Source: CAD feature listing. Evaluate the final solid. Frame: model axes, mm. Face numbers are marked on the shaded views. Coordinates: 2 decimals unless noted, no trailing zeros. Loops run counter-clockwise (first coordinate to the right, second up) from the corner with the lowest first, then second, coordinate; pieces in that order, holes last.
from build123d import *

# Parameters (mm, degrees)
SKETCH1_W                        = 234.95
SKETCH1_H                        = 76.2
EXTRUDE1_DEPTH                   = 12.7
F_1_2_CLEARANCE_HOLE1_AT_2_COUNT = 2
F_1_2_CLEARANCE_HOLE1_AT_2_PITCH = 44.45
F_1_2_CLEARANCE_HOLE1_AT_3_COUNT = 2
F_1_2_CLEARANCE_HOLE1_AT_3_PITCH = 203.2
F_1_2_CLEARANCE_HOLE1_AT_4_COUNT = 2
F_1_2_CLEARANCE_HOLE1_AT_4_PITCH = 208.004909798
SKETCH6_W                        = 171.45
SKETCH6_H                        = 76.2
CUT_EXTRUDE1_DEPTH               = 1.016
F_1_4_20_TAPPED_HOLE1_AT_2_COUNT = 2
F_1_4_20_TAPPED_HOLE1_AT_2_PITCH = 63.5
F_1_4_20_TAPPED_HOLE1_AT_3_COUNT = 2
F_1_4_20_TAPPED_HOLE1_AT_3_PITCH = 127


with BuildPart() as part:
    # Sketch1 → Extrude1 (new body)
    with BuildSketch(Plane.XY):
        Rectangle(SKETCH1_W, SKETCH1_H)
    extrude(amount=EXTRUDE1_DEPTH)

    # Sketch2 → 1/2 Clearance Hole1 (revolve, cut)
    with BuildSketch(Plane(origin=(-101.6, 22.225, 12.7), x_dir=(0, -1, 0), z_dir=(1, 0, 0))):
        Polygon((0, 0), (0, 12.7), (10.16, 12.7), (9.525, 11.969516061), (9.525, 0.730483939), (10.16, 0), align=None)
    f_1_2_clearance_hole1 = revolve(axis=Axis((-101.6, 22.225, 19.05), (0, 0, -1)), mode=Mode.SUBTRACT)

    # 1/2 Clearance Hole1 at 2: 1/2 Clearance Hole1 ×2
    with Locations(*[(0, -i * F_1_2_CLEARANCE_HOLE1_AT_2_PITCH, 0) for i in range(1, F_1_2_CLEARANCE_HOLE1_AT_2_COUNT)]):
        add(f_1_2_clearance_hole1, mode=Mode.SUBTRACT)

    # 1/2 Clearance Hole1 at 3: 1/2 Clearance Hole1 ×2
    with Locations(*[(i * F_1_2_CLEARANCE_HOLE1_AT_3_PITCH, 0, 0) for i in range(1, F_1_2_CLEARANCE_HOLE1_AT_3_COUNT)]):
        add(f_1_2_clearance_hole1, mode=Mode.SUBTRACT)

    # 1/2 Clearance Hole1 at 4: 1/2 Clearance Hole1 ×2
    with Locations(*[Vector(0.976900017, -0.213696879, 0) * (i * F_1_2_CLEARANCE_HOLE1_AT_4_PITCH) for i in range(1, F_1_2_CLEARANCE_HOLE1_AT_4_COUNT)]):
        add(f_1_2_clearance_hole1, mode=Mode.SUBTRACT)

    # Sketch6 → Cut-Extrude1 (cut)
    with BuildSketch(Plane(origin=(0, 0, 0), x_dir=(-1, 0, 0), z_dir=(0, 0, -1))):
        Rectangle(SKETCH6_W, SKETCH6_H)
    extrude(amount=-CUT_EXTRUDE1_DEPTH, mode=Mode.SUBTRACT)

    # Sketch4 → 1/4-20 Tapped Hole1 (revolve, cut)
    with BuildSketch(Plane(origin=(-63.5, 0, 12.7), x_dir=(0, -1, 0), z_dir=(1, 0, 0))):
        Polygon((0, 0), (0, 11.684), (3.81, 11.684), (2.5527, 10.237641802), (2.5527, 1.446358198), (3.81, 0), align=None)
    f_1_4_20_tapped_hole1 = revolve(axis=Axis((-63.5, 0, 19.05), (0, 0, -1)), mode=Mode.SUBTRACT)

    # 1/4-20 Tapped Hole1 at 2: 1/4-20 Tapped Hole1 ×2
    with Locations(*[(i * F_1_4_20_TAPPED_HOLE1_AT_2_PITCH, 0, 0) for i in range(1, F_1_4_20_TAPPED_HOLE1_AT_2_COUNT)]):
        add(f_1_4_20_tapped_hole1, mode=Mode.SUBTRACT)

    # 1/4-20 Tapped Hole1 at 3: 1/4-20 Tapped Hole1 ×2
    with Locations(*[(i * F_1_4_20_TAPPED_HOLE1_AT_3_PITCH, 0, 0) for i in range(1, F_1_4_20_TAPPED_HOLE1_AT_3_COUNT)]):
        add(f_1_4_20_tapped_hole1, mode=Mode.SUBTRACT)


solid = part.part
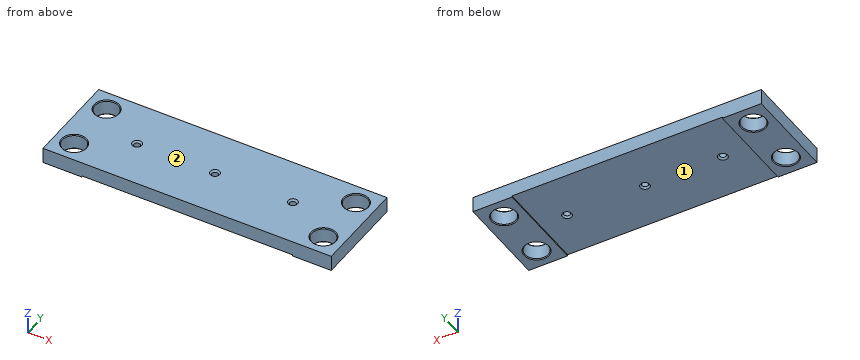
Q1. Draft query along X for the marked faces 1 and 2. Return one class per face: +X half, -X half, draft (parallel to the pull), parting line (faces both ways), or undercut.
Q2. Section B-B, the plane y = 0. Count the separate pieces of the cut face and the enclosed holes in it, plus the area to 3 significant figures.
Q3. Section D-D, the plane x = -101.6. Return the cut outline in (y, z) (3 decimals).
Q4. Contact query for a flat-ended pin moving along its axis: pin 1 Ø23 at (x, y) = (33.5, -16.5) entering from -Z. Output: stop coordinate, or through.
Q5. Section A-A, the plane x = -63.5. Return the cut outline in (y, z), plus the area to 3 significant figures.
Q6. Line query: line 1 along X through (y, z) = (0, 9.25) (3 decimals); line 2 along X through (y, z) = (-22.5, 7.75) (3 decimals); line 3 along Y through (x, z) = (101.6, 6.5). Output: solid intervals per line, ascending.
Q7. Section C-C, the plane z = 8.75. Return the cut outline in (x, y) (3 decimals), plus the area to 3 significant figures.
Derived:
1. face 1: undercut
1. face 2: draft
2. separate pieces: 4
2. enclosed holes: 0
2. area: 2,620 mm2
3. outline: (-38.1, 0) - (-32.385, 0) - (-31.75, 0.73) - (-31.75, 11.97) - (-32.385, 12.7) - (-38.1, 12.7) - close; (-12.7, 0.73) - (-12.065, 0) - (12.065, 0) - (12.7, 0.73) - (12.7, 11.97) - (12.065, 12.7) - (-12.065, 12.7) - (-12.7, 11.97) - close; (31.75, 0.73) - (32.385, 0) - (38.1, 0) - (38.1, 12.7) - (32.385, 12.7) - (31.75, 11.97) - close
4. pin 1: stops at z = 1.02
5. outline: (-38.1, 1.02) - (-3.81, 1.02) - (-2.55, 2.46) - (-2.55, 11.25) - (-3.81, 12.7) - (-38.1, 12.7) - close; (2.55, 2.46) - (3.81, 1.02) - (38.1, 1.02) - (38.1, 12.7) - (3.81, 12.7) - (2.55, 11.25) - close
5. area: 827 mm2
6. line 1: x = -117.475 to -66.053, -60.947 to -2.553, 2.553 to 60.947, 66.053 to 117.475
6. line 2: x = -117.475 to -111.121, -92.079 to 92.079, 111.121 to 117.475
6. line 3: y = -38.1 to -31.75, -12.7 to 12.7, 31.75 to 38.1
7. outline: (-117.475, -38.1) - (117.475, -38.1) - (117.475, 38.1) - (-117.475, 38.1) - close; hole circle Ø19.05 at (-101.6, -22.225); hole circle Ø19.05 at (-101.6, 22.225); hole circle Ø5.105 at (-63.5, 0); hole circle Ø5.105 at (0, 0); hole circle Ø5.105 at (63.5, 0); hole circle Ø19.05 at (101.6, -22.225); hole circle Ø19.05 at (101.6, 22.225)
7. area: 16,700 mm2
